Verification items for the finished model (mm, model axes). Face numbers are marked on the shaded views. A direction names the side the tool comes from. Give positions to 0.01 mm unless a question says otherwise; leave off trailing zeros. Loops run counter-clockwise (first coordinate to the right, second up) from the corner with the lowest first, then second, coordinate; pieces in that order, holes last. Notation, with made-up numbers: (67.5, 0) -> (112.5, 0) arc R32 ccw to (112.5, 30) -> close; hole circle Ø4 at (72.25, 35.25). An arc over 180 degrees is marked (long way). Answer in a Markdown table with one row per item. Add a question column.
Q1. Section check B-B on x = 4.5. Enter the section's corners in (y, z), and give its area (3 significant figures).
Q2. Set-up check for the marked faces 5, 6, 7, 8 and 9: record each of +Z, -Z, +X, -X, +Y, -Y from which the full face is reachable in a straight line by a thin tool's end or side.
Q3. Material ranges on probe 1 along Z at (x, y) = (24.5, 12.25); probe 2 along Z at (x, y) = (21.5, 18.5); probe 3 along Y at (x, z) = (26.75, 8.75), recorded low to high.
Q4. Section check D-D on z = 2. Enter the section's corners in (x, y), and give its area (4 significant figures).
Q5. Gauge pin test, flat ends, axial feed: P1, Ø1.5, axis at x = 2, y = 7, coming from the -Z side; P2, Ø8, axis at x = 5, y = 17, coming from the -Z side; P3, Ø4, axis at x = 1.5, z = 21.5, coming from the +Y side; P4, Ø4.5, axis at y = 13.5, z = 16, coming from the +X side. Record the tip position at first contact, or that the pin passes through.
Q6. Section check C-C on y = 10.75. Enter the section's corners in (x, z), and give its area (3 significant figures).
Q7. Release check for a two-part mould opening along Z. For the marked faces 1, 2, 3 and 4 record: pulls with the +Z half, pulls with the -Z half, needs draft (parallel to the pull), parting line crosses it, or undercut.
Q8. Section check A-A on y = 21.75. Enter the section's corners in (x, z).
```python
from build123d import *

# Parameters (mm, degrees)
BOSS_EXTRUDE1_DEPTH = 25
SKETCH2_W           = 5
SKETCH2_H           = 15
CUT_EXTRUDE1_DEPTH  = 25
SKETCH3_W           = 5
SKETCH3_H           = 5
CUT_EXTRUDE2_DEPTH  = 20
SKETCH4_W           = 5
SKETCH4_H           = 10
CUT_EXTRUDE3_DEPTH  = 10


with BuildPart() as part:
    # Sketch1 → Boss-Extrude1 (new body)
    with BuildSketch(Plane.XY):
        Polygon((0, 0), (30, 0), (30, 25), (20, 25), (5, 10), (0, 10), align=None)
    extrude(amount=BOSS_EXTRUDE1_DEPTH)

    # Sketch2 → Cut-Extrude1 (cut)
    with BuildSketch(Plane(origin=(0, 10, 0), x_dir=(1, 0, 0), z_dir=(0, 1, 0))):
        with Locations((2.5, -12.5)):
            Rectangle(SKETCH2_W, SKETCH2_H)
    extrude(amount=-CUT_EXTRUDE1_DEPTH, mode=Mode.SUBTRACT)

    # Sketch3 → Cut-Extrude2 (cut)
    with BuildSketch(Plane(origin=(0, 25, 0), x_dir=(1, 0, 0), z_dir=(0, 1, 0))):
        Polygon((30, -20), (30, -5), (20, -5), (20, -10), (25, -10), (25, -15), (20, -15), (20, -20), align=None)
        with Locations((17.5, -7.5)):
            Rectangle(SKETCH3_W, SKETCH3_H)
        with Locations((17.5, -17.5)):
            Rectangle(SKETCH3_W, SKETCH3_H)
    extrude(amount=-CUT_EXTRUDE2_DEPTH, mode=Mode.SUBTRACT)

    # Sketch4 → Cut-Extrude3 (cut)
    with BuildSketch(Plane(origin=(25, 0, 0), x_dir=(0, 0, -1), z_dir=(1, 0, 0))):
        with Locations((-12.5, 20)):
            Rectangle(SKETCH4_W, SKETCH4_H)
    extrude(amount=-CUT_EXTRUDE3_DEPTH, mode=Mode.SUBTRACT)


solid = part.part
```
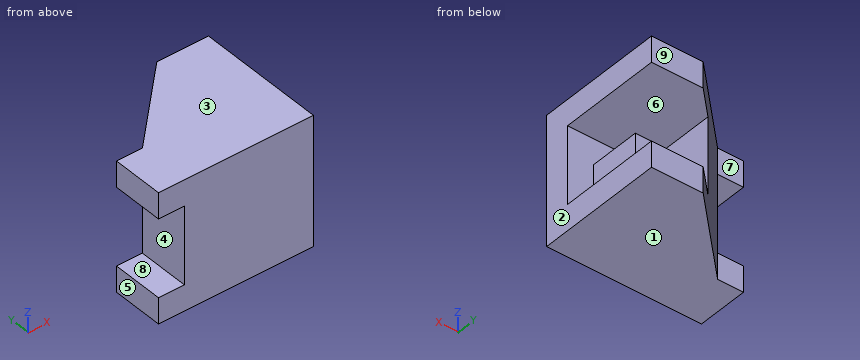
Taken from the geometry:
| question | item | result |
|---|---|---|
| 1 | outline | (0, 0) -> (10, 0) -> (10, 5) -> (0, 5) -> close; (0, 20) -> (10, 20) -> (10, 25) -> (0, 25) -> close |
| 1 | area | 100 mm² |
| 2 | face 5 | +Z, -Z, -X, +Y, -Y |
| 2 | face 6 | +X, +Y |
| 2 | face 7 | +Z, -Z, -X, +Y |
| 2 | face 8 | -X, +Y, -Y |
| 2 | face 9 | +Z, -Z, +X, -X, +Y |
| 3 | probe 1 | z = 0 to 5, 10 to 15, 20 to 25 |
| 3 | probe 2 | z = 0 to 5, 20 to 25 |
| 3 | probe 3 | y = 0 to 5 |
| 4 | outline | (0, 0) -> (30, 0) -> (30, 25) -> (20, 25) -> (5, 10) -> (0, 10) -> close |
| 4 | area | 562.5 mm² |
| 5 | P1 | stops at z = 0 |
| 5 | P2 | passes through |
| 5 | P3 | stops at y = 10 |
| 5 | P4 | stops at x = 25 |
| 6 | outline | (5.75, 0) -> (30, 0) -> (30, 5) -> (15, 5) -> (15, 10) -> (25, 10) -> (25, 15) -> (15, 15) -> (15, 20) -> (30, 20) -> (30, 25) -> (5.75, 25) -> close |
| 6 | area | 431 mm² |
| 7 | face 1 | pulls with the -Z half |
| 7 | face 2 | needs draft |
| 7 | face 3 | pulls with the +Z half |
| 7 | face 4 | undercut |
| 8 | outline | (16.75, 0) -> (30, 0) -> (30, 5) -> (16.75, 5) -> close; (16.75, 20) -> (30, 20) -> (30, 25) -> (16.75, 25) -> close |
